The model under review builds one solid part; all positions refer to its coordinate system, in mm. A direction names the side the tool comes from. Coordinates: 2 decimals unless noted, no trailing zeros. Order: outer loops, then holes, each group sorted by start corner. A loop starts at its lowest first (then second) coordinate and runs counter-clockwise, first axis right, second up. Notation, with made-up numbers: (58, -19) -> (92, -19) arc R25 cw to (92, 2) -> close; hole circle Ø8 at (-24.5, -33). An arc over 180 degrees is marked (long way). Use CSV: the item, a comma, the result in double quotes. Start each with the question number.
```python
from build123d import *

# Parameters (mm, degrees)
SKETCH1_W           = 12.8
SKETCH1_H           = 5.8
BOSS_EXTRUDE1_DEPTH = 6.5
SKETCH2_R           = 1.025
CUT_EXTRUDE1_DEPTH  = 11.80971785
SKETCH3_W           = 0.8
SKETCH3_H           = 0.5
BOSS_EXTRUDE2_DEPTH = 2.4
BOSS_EXTRUDE3_DEPTH = 1.5


with BuildPart() as part:
    # Sketch1 → Boss-Extrude1 (new body)
    with BuildSketch(Plane(origin=(0, 0, 0), x_dir=(1, 0, 0), z_dir=(0, 1, 0))):
        Rectangle(SKETCH1_W, SKETCH1_H)
    extrude(amount=BOSS_EXTRUDE1_DEPTH)

    # Sketch2 → Cut-Extrude1 (cut, through all)
    with BuildSketch(Plane.XY.offset(2.9)):
        with Locations((-3.25, 1.425)):
            Circle(SKETCH2_R)
        with Locations((3.25, 1.425)):
            Circle(SKETCH2_R)
        Polygon((-6.4, 0.2), (-4.25, 0.2), (-4.134529946, 0), (-6.4, 0), align=None)
        Polygon((4.134529946, 0), (6.4, 0), (6.4, 0.2), (4.25, 0.2), align=None)
        Polygon((2.365470054, 0), (2.25, 0.2), (-2.25, 0.2), (-2.365470054, 0), align=None)
    extrude(amount=-CUT_EXTRUDE1_DEPTH, mode=Mode.SUBTRACT)

    # Sketch3 → Boss-Extrude2 (add)
    with BuildSketch(Plane.XZ.offset(-0.2)):
        Rectangle(SKETCH3_W, SKETCH3_H)
        with Locations((5.08, 0)):
            Rectangle(SKETCH3_W, SKETCH3_H)
        with Locations((-5.08, 0)):
            Rectangle(SKETCH3_W, SKETCH3_H)
    extrude(amount=BOSS_EXTRUDE2_DEPTH)

    # Sketch4 → Boss-Extrude3 (add, symmetric)
    with BuildSketch(Plane.XY):
        with BuildLine():
            Line((-5.8, 6.5), (-5.8, 6.6))
            ThreePointArc((-5.8, 6.6), (-5.672582553, 6.969683285), (-5.344447564, 7.182352901))
            Line((-5.344447564, 7.182352901), (7.627776218, 10.4))
            Line((7.627776218, 10.4), (7.7, 10.108823549))
            Line((7.7, 10.108823549), (-5.272223782, 6.891176451))
            ThreePointArc((-5.272223782, 6.891176451), (-5.436291276, 6.784841642), (-5.5, 6.6))
            Line((-5.5, 6.6), (-5.5, 6.5))
            Line((-5.5, 6.5), (-5.8, 6.5))
        make_face()
    extrude(amount=BOSS_EXTRUDE3_DEPTH, both=True)


solid = part.part
```
Q1. Add section C-C, the plane x = -1. State the section outline as (y, z) points, then the cut area to 3 significant figures.
Q2. Clearance check with flat-ended pins moving along their axes: pin 1 Ø1.2 at (x, y) = (-2.5, 9.5) entering from -Z; pin 2 Ø3 at (y, z) = (3, 0) entering from +X; pin 3 Ø0.5 at (x, z) = (-3, 1) entering from -Y; pin 4 Ø0.9 at (x, y) = (0, -0.5) entering from -Z. State where each tip first meets the part, or that it passes through.
Q3. Draft analysis for pull direction Y (two halves, no side actions). For faces 1 (the flat face through (-3, 0, 0)), 2 (the flat face through (5, -1, -0.25)), 3 (the flat face through (1.3, 8.52, 0.02)), state which applies: +Y half, -Y half, draft (parallel to the pull), parting line (faces both ways), or undercut.
Q4. Add section B-B, the plane x = 3.5. State the section outline as (y, z) points.
Q5. For faces 4 (the flat face through (0, 3, 2.9)), 5 (the flat face through (6.4, 3, 0)), list the 3-axis set-ups (+Z, -Z, +X, -X, +Y, -Y) from which the entire face can be reached by the end or side of a thin tool; tool diameter is ignored.
Q6. Add section D-D, the plane y = 4. State the section outline as (x, z) points, then the cut area to 3 significant figures.
Q7. To check wall thickness, follow probe 1 along Y at (x, z) = (-3.25, 1.6); probe 2 along X at (y, z) = (2.25, -2.45); probe 3 along Y at (x, z) = (-3.25, -0.3). State the ranges of each line that lie inside material, in increasing order.
Answer block:
1,outline,"(0.2, -2.9) -> (6.5, -2.9) -> (6.5, 2.9) -> (0.2, 2.9) -> close; (7.95, -1.5) -> (8.26, -1.5) -> (8.26, 1.5) -> (7.95, 1.5) -> close"
1,area,"37.5 mm²"
2,pin 1,"passes through"
2,pin 2,"stops at x = 6.4"
2,pin 3,"stops at y = 0"
2,pin 4,"stops at z = -0.25"
3,face 1,"-Y half"
3,face 2,"draft"
3,face 3,"undercut"
4,outline,"(0, -2.9) -> (0.43, -2.9) -> (0.43, 2.9) -> (0, 2.9) -> close; (2.42, -2.9) -> (6.5, -2.9) -> (6.5, 2.9) -> (2.42, 2.9) -> close; (9.07, -1.5) -> (9.38, -1.5) -> (9.38, 1.5) -> (9.07, 1.5) -> close"
5,face 4,"+Z, +X, -X, +Y, -Y"
5,face 5,"+Z, -Z, +X, -Y"
6,outline,"(-6.4, -2.9) -> (6.4, -2.9) -> (6.4, 2.9) -> (-6.4, 2.9) -> close"
6,area,"74.2 mm²"
7,probe 1,"y = 0 to 0.4, 2.45 to 6.5"
7,probe 2,"x = -6.4 to -3.86, -2.64 to 2.64, 3.86 to 6.4"
7,probe 3,"y = 0 to 0.4, 2.45 to 6.5, 7.39 to 7.7"
